from build123d import *

# Parameters (mm, degrees)
BOSS_EXTRUDE1_DEPTH      = 43
BOSS_EXTRUDE2_DEPTH      = 11
BOSS_EXTRUDE2_DEPTH_BACK = 11
CUT_EXTRUDE1_DEPTH       = 87.401678224
CUT_EXTRUDE1_DEPTH_BACK  = 87.401678224
SKETCH3_R                = 5.25
SKETCH3_R_2              = 5


with BuildPart() as part:
    # Sketch1 → Boss-Extrude1 (new body)
    with BuildSketch(Plane.XY):
        with BuildLine():
            Line((-6.5, 9), (-6.5, -9))
            Line((-6.5, -9), (-6.119061554, -9))
            Line((-6.119061554, -9), (-6.119061554, -22))
            Line((-6.119061554, -22), (-12.119061554, -22))
            Line((-12.119061554, -22), (-12.119061554, -8.960698063))
            Line((-12.119061554, -8.960698063), (-12.5, -8.960698063))
            Line((-12.5, -8.960698063), (-12.5, 7.308339657))
            ThreePointArc((-12.5, 7.308339657), (-11.36319561, 11.939080805), (-8.211247284, 15.51697258))
            ThreePointArc((-8.211247284, 15.51697258), (0, 18.0924797), (8.211247284, 15.51697258))
            ThreePointArc((8.211247284, 15.51697258), (11.36319561, 11.939080805), (12.5, 7.308339657))
            Line((12.5, 7.308339657), (12.5, -8.989240444))
            Line((12.5, -8.989240444), (12.119061554, -8.989240444))
            Line((12.119061554, -8.989240444), (12.119061554, -22))
            Line((12.119061554, -22), (6.119061554, -22))
            Line((6.119061554, -22), (6.119061554, -9))
            Line((6.119061554, -9), (6.5, -9))
            Line((6.5, -9), (6.5, 9))
            ThreePointArc((6.5, 9), (0, 12.0924797), (-6.5, 9))
        make_face()
    extrude(amount=BOSS_EXTRUDE1_DEPTH)

    # Sketch2 → Boss-Extrude2 (add, two sides: drawn at the far end of the back side and taken through both)
    with BuildSketch(Plane(origin=(0, 0, 0), x_dir=(1, 0, 0), z_dir=(0, 1, 0)).offset(-BOSS_EXTRUDE2_DEPTH_BACK)):
        with BuildLine():
            Line((-20.5, -81), (-20.5, -47.820060952))
            ThreePointArc((-20.5, -47.820060952), (-18.187988462, -41.966506434), (-12.5, -39.272757167))
            Line((-12.5, -39.272757167), (-6.5, -39.272757167))
            Line((-6.5, -39.272757167), (-6.5, -43))
            Line((-6.5, -43), (-14.5, -45.836759656))
            Line((-14.5, -45.836759656), (-14.5, -81))
            Line((-14.5, -81), (-20.5, -81))
        make_face()
        with BuildLine():
            Line((6.5, -39.272757167), (12.5, -39.272757167))
            ThreePointArc((12.5, -39.272757167), (18.187988462, -41.966506434), (20.5, -47.820060952))
            Line((20.5, -47.820060952), (20.5, -81))
            Line((20.5, -81), (14.5, -81))
            Line((14.5, -81), (14.5, -45.836759656))
            Line((14.5, -45.836759656), (6.5, -43))
            Line((6.5, -43), (6.5, -39.272757167))
        make_face()
    extrude(amount=BOSS_EXTRUDE2_DEPTH + BOSS_EXTRUDE2_DEPTH_BACK)

    # Sketch3 → Cut-Extrude1 (cut, two sides: drawn at the far end of the back side and taken through both)
    with BuildSketch(Plane(origin=(0, 0, 0), x_dir=(0, 0, -1), z_dir=(1, 0, 0)).offset(-CUT_EXTRUDE1_DEPTH_BACK)):
        with Locations(Location((-14, -14, 0), (0, 0, 72.247209838))):
            Circle(SKETCH3_R)
        with Locations((-69, 0)):
            Circle(SKETCH3_R_2)
        Polygon((-5.082033537, -23.71409096), (2.018266343, -14.692533465), (6.529045091, -36.912295444), align=None)
        with BuildLine():
            Line((-69, 11), (-69, 14.018852996))
            Line((-69, 14.018852996), (-85.29582804, 14.018852996))
            Line((-85.29582804, 14.018852996), (-85.29582804, -20.343414377))
            Line((-85.29582804, -20.343414377), (-69, -16.597000701))
            Line((-69, -16.597000701), (-69, -11))
            ThreePointArc((-69, -11), (-80, 0), (-69, 11))
        make_face()
    extrude(amount=CUT_EXTRUDE1_DEPTH + CUT_EXTRUDE1_DEPTH_BACK, mode=Mode.SUBTRACT)


solid = part.part
Design review of the part built by this model. Coordinates are the model's own, in mm. A direction names the side the tool comes from. Give positions to 0.01 mm unless a question says otherwise; leave off trailing zeros. Order: outer loops, then holes, each group sorted by start corner. A loop starts at its lowest first (then second) coordinate and runs counter-clockwise, first axis right, second up.
1. Add section A-A, the plane y = -14. State the section outline as (x, z) points.
Solution:
outline: (-12.12, 0) - (-6.12, 0) - (-6.12, 8.75) - (-12.12, 8.75) - close; (-12.12, 19.25) - (-6.12, 19.25) - (-6.12, 43) - (-12.12, 43) - close; (6.12, 0) - (12.12, 0) - (12.12, 8.75) - (6.12, 8.75) - close; (6.12, 19.25) - (12.12, 19.25) - (12.12, 43) - (6.12, 43) - close
2. For pin 1 Ø6.5 at (x, y) = (9, -12.5) entering from +Z; pin 2 Ø10.5 at (y, z) = (-14, 13.5) entering from +X; pin 3 Ø4.5 at (x, y) = (-5.5, 15) entering from +Z, all flat-tipped, find the tip position at first contact; note any pin that passes through.
Solution:
pin 1: stops at z = 44.91
pin 2: stops at x = 12.5
pin 3: stops at z = 43
3. Add section C-C, the plane z = 55.5. State the section outline as (x, y) points, then the cut area to 3 significant figures.
Solution:
outline: (-20.5, -11) - (-14.5, -11) - (-14.5, 11) - (-20.5, 11) - close; (14.5, -11) - (20.5, -11) - (20.5, 11) - (14.5, 11) - close
area: 264 mm2
4. Add section D-D, the plane z = 70. State the section outline as (x, y) points.
Solution:
outline: (-20.5, -10.95) - (-14.5, -10.95) - (-14.5, -4.9) - (-20.5, -4.9) - close; (-20.5, 4.9) - (-14.5, 4.9) - (-14.5, 10.95) - (-20.5, 10.95) - close; (14.5, -10.95) - (20.5, -10.95) - (20.5, -4.9) - (14.5, -4.9) - close; (14.5, 4.9) - (20.5, 4.9) - (20.5, 10.95) - (14.5, 10.95) - close
5. To check wall thickness, follow L1, parallel to Y at x = 17, z = 69; L2, parallel to Z at x = 10.25, y = -14; L3, parallel to X at y = -2.5, z = 12. State the ranges of each line that lie inside material, in increasing order.
Solution:
L1: y = -11 to -5, 5 to 11
L2: z = 0 to 8.75, 19.25 to 43
L3: x = -12.5 to -6.5, 6.5 to 12.5
6. Add section B-B, the plane z = 14. State the section outline as (x, y) points.
Solution:
outline: (-12.5, -8.75) - (-6.5, -8.75) - (-6.5, 9) arc R8.38 cw to (6.5, 9) - (6.5, -8.75) - (12.5, -8.75) - (12.5, 7.31) arc R10 ccw to (8.21, 15.52) arc R14.38 ccw to (-8.21, 15.52) arc R10 ccw to (-12.5, 7.31) - close; (-12.12, -22) - (-6.12, -22) - (-6.12, -19.25) - (-12.12, -19.25) - close; (6.12, -22) - (12.12, -22) - (12.12, -19.25) - (6.12, -19.25) - close
7. Mouldability with a two-part tool opening along X and no side actions: class faces 1 (the flat face through (-10.444, -0.154, 44.399)), 2 (the cylindrical face through (9.265, -18.942, 12.228)), 3 (the flat face through (10.56, -0.15, 44.44)), 4 (the flat face through (20.5, -0.2, 63.7)) as +X half, -X half, draft (parallel to the pull), parting line (faces both ways), or undercut.
Solution:
face 1: undercut
face 2: draft
face 3: undercut
face 4: +X half
8. Tool access review of faces 5 (the flat face through (-12.5, -1, 19)), 6 (the cylindrical face through (-9.35, -8.75, 13.98)): name each direction out of +Z, -Z, +X, -X, +Y, -Y from which nothing blocks a thin tool from reaching the whole face with its end or side.
Solution:
face 5: -Z, -X, +Y, -Y
face 6: +X, -X
